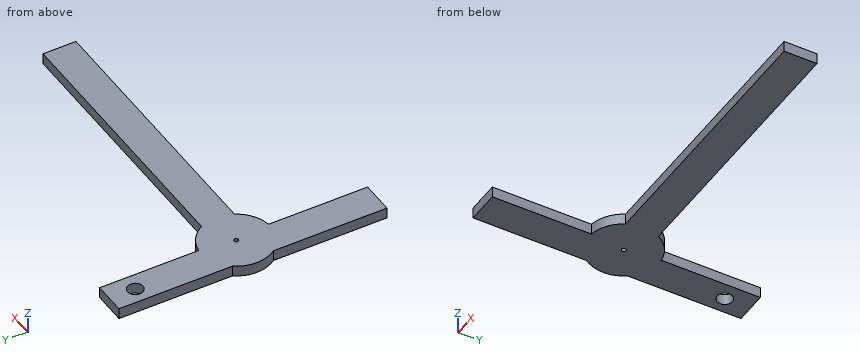
Autodesk Inventor part; units mm, degrees
ref_plane "YZ Plane" through (0, 0, 0) normal (1, 0, 0) x (0, 1, 0)
ref_plane "XZ Plane" through (0, 0, 0) normal (0, 1, 0) x (-1, 0, 0)
ref_plane "XY Plane" through (0, 0, 0) normal (0, 0, 1) x (1, 0, 0)
sketch "Boceto1" plane through (0, 0, 0) normal (0, 0, 1) x (1, 0, 0)
  line L0 (0, -51.6726) -> (0, 0)
  line L1 (0, 0) -> (15, 0)
  line L2 (15, 0) -> (15, -45.1255)
  circle A0 centre (7.2527, -11.7) radius 3.5
  arc A1 (0, -51.6726) -> (0, -70.3274) centre (13, -61) ccw
  line L3 (27.1333, -53.5) -> (150, -53.5)
  line L4 (150, -53.5) -> (150, -68.5)
  line L5 (150, -68.5) -> (27.1333, -68.5)
  line L6 (15, -76.8745) -> (15, -122)
  line L7 (15, -122) -> (0, -122)
  line L8 (0, -122) -> (0, -70.3274)
  arc A2 (15, -76.8745) -> (27.1333, -68.5) centre (13, -61) ccw
  arc A3 (27.1333, -53.5) -> (15, -45.1255) centre (13, -61) ccw
  circle A4 centre (13, -61) radius 1
  point P0 (0, -70.3274)
  point P1 (15, -76.8745)
  dimension "d0" = 2
extrude "Extrusión1" add sketch "Boceto1" along normal blind 5
properties part number "P3"
Here's how the part is built. I have some questions about the finished solid (model axes, mm). Give positions to 0.01 mm unless a question says otherwise; leave off trailing zeros. Order: outer loops, then holes, each group sorted by start corner. A loop starts at its lowest first (then second) coordinate and runs counter-clockwise, first axis right, second up. Notation, with made-up numbers: (8.5, -39.75) - (23.5, -39.75) arc R20 ccw to (23.5, -13.75) - close; hole circle Ø6 at (25, 30). An arc over 180 degrees is marked (long way). Answer as a JSON object with one key per item and string values. Group by question number.
Item 1: If we section it at A-A on y = -11.7: Please give me the cut outline in (x, z).
Item 2: Please list where these lines run through material, in increasing order: probe 1 along Y at (x, z) = (13, 2.7); probe 2 along X at (y, z) = (-83, 1); probe 3 along Y at (x, z) = (82, 3.5).
Item 3: If we section it at D-D on y = -26: Please give me the cut outline in (x, z), and give its area (3 significant figures).
Item 4: If we section it at C-C on x = 81.5: Please give me the cut outline in (y, z).
Item 5: If we section it at B-B on z = 1.75: Please give me the cut outline in (x, y), and give its area (3 significant figures).
Item 6: For P1, Ø3, axis at y = -16.5, z = 3.5, coming from the +X side; P2, Ø2.5, axis at x = 84.5, z = 3, coming from the +Y side; P3, Ø3, axis at x = 23.5, y = -76, coming from the -Z side (1 decimal); P4, Ø2.5, axis at y = -96, z = 2, coming from the -X side, each with a flat end and sliding along its axis, tell me the tip position at first contact or that it passes through.
Result set:
{
 "1": {"outline": "(0, 0) - (3.75, 0) - (3.75, 5) - (0, 5) - close; (10.75, 0) - (15, 0) - (15, 5) - (10.75, 5) - close"},
 "2": {"probe 1": "-122 to -62, -60 to 0", "probe 2": "0 to 15", "probe 3": "-68.5 to -53.5"},
 "3": {"outline": "(0, 0) - (15, 0) - (15, 5) - (0, 5) - close", "area": "75.0 mm²"},
 "4": {"outline": "(-68.5, 0) - (-53.5, 0) - (-53.5, 5) - (-68.5, 5) - close"},
 "5": {"outline": "(0, -122) - (15, -122) - (15, -76.87) arc R16 ccw to (27.13, -68.5) - (150, -68.5) - (150, -53.5) - (27.13, -53.5) arc R16 ccw to (15, -45.13) - (15, 0) - (0, 0) - (0, -51.67) arc R16 ccw to (0, -70.33) - close; hole circle Ø7 at (7.25, -11.7); hole circle Ø2 at (13, -61)", "area": "3,990 mm²"},
 "6": {"P1": "x = 15", "P2": "y = -53.5", "P3": "through", "P4": "x = 0"}
}
